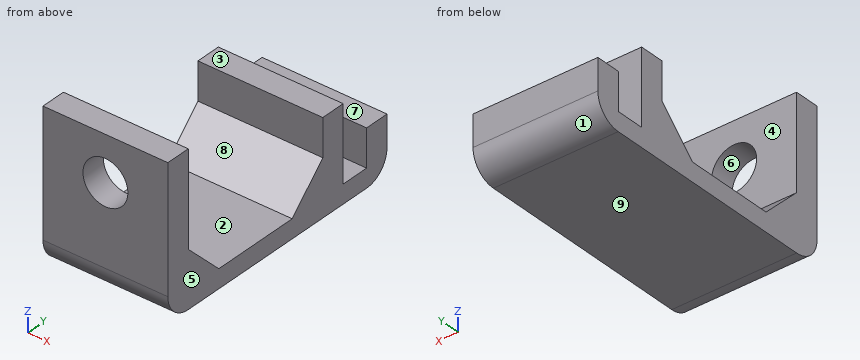
from build123d import *

# Parameters (mm, degrees)
BOSS_EXTRUDE1_DEPTH     = 5
CHAMFER1_SIZE           = 3
SKETCH2_R               = 1.8
CUT_EXTRUDE1_DEPTH      = 3
CUT_EXTRUDE1_DEPTH_BACK = 3
FILLET1_R               = 2


with BuildPart() as part:
    # Sketch1 → Boss-Extrude1 (new body, symmetric)
    with BuildSketch(Plane(origin=(0, 0, 0), x_dir=(0, 0, -1), z_dir=(1, 0, 0))):
        Polygon((-5.25, -8.75), (-5.25, -10.75), (6.75, -10.75), (6.75, 10.75), (2.25, 10.75), (2.25, 8.75), (5.25, 8.75), (5.25, 6.45), (-0.75, 6.45), (-0.75, 4.45), (5.25, 4.45), (5.25, -8.75), align=None)
    extrude(amount=BOSS_EXTRUDE1_DEPTH, both=True)

    # Chamfer1
    chamfer1_edges = [part.edges().sort_by_distance(p)[0] for p in [
        (0, -8.75, -5.25),
        (0, 4.45, -5.25),
    ]]
    chamfer(chamfer1_edges, length=CHAMFER1_SIZE)

    # Sketch2 → Cut-Extrude1 (cut, two sides)
    with BuildSketch(Plane(origin=(0, -8.75, 0), x_dir=(1, 0, 0), z_dir=(0, 1, 0))) as cut_extrude1_sk:
        with Locations((0, -1.65)):
            Circle(SKETCH2_R)
    extrude(amount=CUT_EXTRUDE1_DEPTH, mode=Mode.SUBTRACT)
    extrude(cut_extrude1_sk.sketch, amount=-CUT_EXTRUDE1_DEPTH_BACK, mode=Mode.SUBTRACT)

    # Fillet1
    fillet1_edges = [part.edges().sort_by_distance(p)[0] for p in [
        (0, 10.75, -6.75),
        (0, -10.75, -6.75),
    ]]
    fillet(fillet1_edges, radius=FILLET1_R)


solid = part.part
Input: part model. Units: mm. Frame: model coordinates. Face numbers are marked on the shaded views. A direction names the side the tool comes from. Give positions to 0.01 mm unless a question says otherwise; leave off trailing zeros. Order: outer loops, then holes, each group sorted by start corner. A loop starts at its lowest first (then second) coordinate and runs counter-clockwise, first axis right, second up. Notation, with made-up numbers: (12, -22) -> (32, -22) arc R11 ccw to (32, -10) -> close; hole circle Ø2 at (12.25, 88). An arc over 180 degrees is marked (long way). Use one line per item in the form item = value.
1) Section A-A, the plane z = -2.5. Return loops of the section in (x, y), and give its area (3 significant figures).
Response values:
outline = (-5, -10.75) -> (5, -10.75) -> (5, -8.5) -> (-5, -8.5) -> close; (-5, 4.2) -> (5, 4.2) -> (5, 6.45) -> (-5, 6.45) -> close; (-5, 8.75) -> (5, 8.75) -> (5, 10.75) -> (-5, 10.75) -> close
area = 65.0 mm^2
2) Line query: probe 1 along Y at (x, z) = (2.5, -1.5); probe 2 along Y at (x, z) = (2.25, -5); probe 3 along Y at (x, z) = (-3, -3). Output: solid intervals per line, ascending.
Response values:
probe_1 = -10.75 to -8.75, 4.45 to 6.45
probe_2 = -10.73 to -6, 1.7 to 6.45, 8.75 to 10.73
probe_3 = -10.75 to -8, 3.7 to 6.45, 8.75 to 10.75
3) Section C-C, the plane z = 1.65. Return loops of the section in (x, y), and give its area (3 significant figures).
Response values:
outline = (-5, -10.75) -> (-1.8, -10.75) -> (-1.8, -8.75) -> (-5, -8.75) -> close; (1.8, -10.75) -> (5, -10.75) -> (5, -8.75) -> (1.8, -8.75) -> close
area = 12.8 mm^2
4) Section D-D, the plane y = -9.25. Return loops of the section in (x, z), and give its area (3 significant figures).
Response values:
outline = (-5, -6.69) -> (5, -6.69) -> (5, 5.25) -> (-5, 5.25) -> close; hole circle Ø3.6 at (0, 1.65)
area = 109 mm^2
5) Mould query, pull axis Y, two halves, no side actions, for the marked faces 1, 2, 3 and 4. Classes: pulls with the +Y half, pulls with the -Y half, needs draft (parallel to the pull), parting line crosses it, or undercut.
Response values:
face_1 = pulls with the +Y half
face_2 = undercut
face_3 = needs draft
face_4 = undercut
6) Section B-B, the plane x = 0. Return loops of the section in (y, z).
Response values:
outline = (-10.75, -4.75) arc R2 ccw to (-8.75, -6.75) -> (8.75, -6.75) arc R2 ccw to (10.75, -4.75) -> (10.75, -2.25) -> (8.75, -2.25) -> (8.75, -5.25) -> (6.45, -5.25) -> (6.45, 0.75) -> (4.45, 0.75) -> (4.45, -2.25) -> (1.45, -5.25) -> (-5.75, -5.25) -> (-8.75, -2.25) -> (-8.75, -0.15) -> (-10.75, -0.15) -> close; (-10.75, 3.45) -> (-8.75, 3.45) -> (-8.75, 5.25) -> (-10.75, 5.25) -> close
7) Reachability of the marked faces 5, 6, 7, 8 and 9 from +Z, -Z, +X, -X, +Y, -Y: full face, straight path, thin tool, end or side. Return the list, or none.
Response values:
face_5 = +Z, -Z, +X, +Y, -Y
face_6 = -Y
face_7 = +Z, +X, -X, +Y
face_8 = +Z, +X, -X
face_9 = -Z, +X, -X, +Y, -Y
8) First-contact query: pin 1 Ø6 at (x, y) = (-1.5, 7.5) entering from +Z; pin 2 Ø2 at (x, z) = (-2, 3) entering from +Y; pin 3 Ø0.7 at (x, y) = (1.5, 7) entering from +Z. Flat tips, straight axial feed; report the tip coordinate or a pass-through.
Response values:
pin_1 = 0.75
pin_2 = -8.75
pin_3 = -5.25
